```python
from build123d import *

# Parameters (mm, degrees)
BOSS_EXTRUDE1_DEPTH = 508
CUT_EXTRUDE1_DEPTH  = 508
BOSS_EXTRUDE2_DEPTH = 508
BOSS_EXTRUDE3_DEPTH = 635
CUT_EXTRUDE3_DEPTH  = 1016
CUT_EXTRUDE6_DEPTH  = 508
CUT_EXTRUDE7_DEPTH  = 1016
CUT_EXTRUDE8_DEPTH  = 1016
CUT_EXTRUDE9_DEPTH  = 1016
CUT_EXTRUDE10_DEPTH = 2092.737749488
SKETCH11_W          = 6.35
SKETCH11_H          = 822.114235363
BOSS_EXTRUDE4_DEPTH = 76.2
SKETCH12_W          = 6.35
SKETCH12_H          = 1181.577860321
BOSS_EXTRUDE5_DEPTH = 81.28


with BuildPart() as part:
    # Sketch1 → Boss-Extrude1 (new body)
    with BuildSketch(Plane(origin=(0, 0, 0), x_dir=(1, 0, 0), z_dir=(0, 1, 0))):
        Polygon((0, 1066.8), (0, 0), (279.4, 0), (457.2, 1066.8), align=None)
    boss_extrude1 = extrude(amount=BOSS_EXTRUDE1_DEPTH)

    # Sketch2 → Cut-Extrude1 (cut)
    with BuildSketch(Plane.ZY):
        Polygon((0, 0), (-1066.8, 508), (-1066.8, 732.672417782), (0, 732.672417782), align=None)
    cut_extrude1 = extrude(amount=-CUT_EXTRUDE1_DEPTH, mode=Mode.SUBTRACT)

    # Sketch3 → Boss-Extrude2 (add)
    with BuildSketch(Plane.XZ):
        Polygon((0, -1066.8), (0, -1854.2), (609.6, -1854.2), (457.2, -1066.8), align=None)
    boss_extrude2 = extrude(amount=-BOSS_EXTRUDE2_DEPTH)

    # Mirror1: Boss-Extrude1 across plane
    add(boss_extrude1.mirror(Plane(origin=(0, 508, -1066.8), x_dir=(0, 0, 1), z_dir=(1, 0, 0))))

    # Mirror1 2: Cut-Extrude1 across plane
    add(cut_extrude1.mirror(Plane(origin=(0, 508, -1066.8), x_dir=(0, 0, 1), z_dir=(1, 0, 0))), mode=Mode.SUBTRACT)


with BuildPart() as body_2:
    # Sketch4 → Boss-Extrude3 (new body)
    with BuildSketch(Plane.XZ):
        Polygon((279.4, 0), (758.024602406, -943.929756814), (824.163316724, -1854.2), (609.6, -1854.2), (473.605368522, -1854.2), (229.324151542, -858.00394067), align=None)
    boss_extrude3 = extrude(amount=-BOSS_EXTRUDE3_DEPTH)

    # Sketch5 → Cut-Extrude3 (cut)
    with BuildSketch(Plane(origin=(158.02566363, 112.959299077, 80.127753023), x_dir=(-0.31022668993908165, -0.22175505323400505, 0.924437178619848), z_dir=(-0.7520567447205982, -0.5375823192171424, -0.38133437136635806))):
        Polygon((-393.664649125, 703.625608499), (953.241894052, -176.928807588), (-1326.842790058, -923.556364957), (-2274.788319735, -628.326732027), (-2325.528348512, 172.375821483), align=None)
    cut_extrude3 = extrude(amount=-CUT_EXTRUDE3_DEPTH, mode=Mode.SUBTRACT)

    # Sketch6 → Cut-Extrude6 (cut)
    with BuildSketch(Plane(origin=(397.94007399, 254.27896004, 77.020659482), x_dir=(0.13564130705663138, 0.08667317707163243, -0.9869595717131874), z_dir=(0.8316697136780645, 0.5314270256083374, 0.16096833167962543))):
        Polygon((1082.533011894, 1261.854611528), (2538.800510351, 767.688534421), (2437.604130324, -1113.046367909), (306.999460867, -1023.580096849), align=None)
    cut_extrude6 = extrude(amount=CUT_EXTRUDE6_DEPTH, mode=Mode.SUBTRACT)

    # Sketch7 → Cut-Extrude7 (cut)
    with BuildSketch(Plane(origin=(0, 0, 0), x_dir=(1, 0, 0), z_dir=(0, 0.9028605188239303, 0.4299335803923477))):
        Polygon((0, 1181.577860321), (0, 0), (1197.045935399, 0), (1543.879463505, 955.927792479), (976.352766556, 2301.292030359), align=None)
    cut_extrude7 = extrude(amount=CUT_EXTRUDE7_DEPTH, mode=Mode.SUBTRACT)

    # Sketch8 → Cut-Extrude8 (cut)
    with BuildSketch(Plane(origin=(382.681643927, 161.632761359, 74.067414954), x_dir=(0.1616973556962576, 0.06829590736935992, -0.9844742933146776), z_dir=(0.9068988908525647, 0.38304573613058523, 0.1755288175843677))):
        Polygon((1197.556798458, 999.143883777), (2455.295967915, 323.49765858), (2410.705423203, -956.043074474), (776.288597468, -956.043074474), (430.351182168, -503.275200855), align=None)
    cut_extrude8 = extrude(amount=CUT_EXTRUDE8_DEPTH, mode=Mode.SUBTRACT)

    # Sketch9 → Cut-Extrude9 (cut)
    with BuildSketch(Plane(origin=(0, 508, 0), x_dir=(1, 0, 0), z_dir=(0, 1, 0))):
        Polygon((351.522364305, 2301.225932819), (1863.401978722, 1800.09916747), (1313.944223798, 629.194662402), (-286.938271333, 375.015467974), (-444.004316346, 1364.25568729), align=None)
    cut_extrude9 = extrude(amount=CUT_EXTRUDE9_DEPTH, mode=Mode.SUBTRACT)


with BuildPart() as part_1:
    add(part.part)

    # Mirror1 3: Boss-Extrude2, Boss-Extrude3 across plane
    add(boss_extrude2.mirror(Plane(origin=(0, 508, -1066.8), x_dir=(0, 0, 1), z_dir=(1, 0, 0))))
    add(boss_extrude3.mirror(Plane(origin=(0, 508, -1066.8), x_dir=(0, 0, 1), z_dir=(1, 0, 0))))

    # Mirror1 4: Cut-Extrude3, Cut-Extrude6, Cut-Extrude7, Cut-Extrude8, Cut-Extrude9 across plane
    add(cut_extrude3.mirror(Plane(origin=(0, 508, -1066.8), x_dir=(0, 0, 1), z_dir=(1, 0, 0))), mode=Mode.SUBTRACT)
    add(cut_extrude6.mirror(Plane(origin=(0, 508, -1066.8), x_dir=(0, 0, 1), z_dir=(1, 0, 0))), mode=Mode.SUBTRACT)
    add(cut_extrude7.mirror(Plane(origin=(0, 508, -1066.8), x_dir=(0, 0, 1), z_dir=(1, 0, 0))), mode=Mode.SUBTRACT)
    add(cut_extrude8.mirror(Plane(origin=(0, 508, -1066.8), x_dir=(0, 0, 1), z_dir=(1, 0, 0))), mode=Mode.SUBTRACT)
    add(cut_extrude9.mirror(Plane(origin=(0, 508, -1066.8), x_dir=(0, 0, 1), z_dir=(1, 0, 0))), mode=Mode.SUBTRACT)


with BuildPart() as cut_extrude10_tool:
    # Sketch10 → Cut-Extrude10 (new, through all)
    with BuildSketch(Plane(origin=(0, 0, 0), x_dir=(0, 0, -1), z_dir=(1, 0, 0))):
        Polygon((2306.148998717, 875.535830554), (458.236130604, 1137.326156156), (-514.568333215, 141.183628961), (336.70111329, -1596.655316262), (2036.802708671, -1025.71271333), (2740.096775658, -499.622195383), align=None)
    extrude(amount=CUT_EXTRUDE10_DEPTH)


with BuildPart() as part_2:
    add(part_1.part)

    # Cut-Extrude10: cut by cut_extrude10_tool
    add(cut_extrude10_tool.part, mode=Mode.SUBTRACT)

    # Sketch11 → Boss-Extrude4 (add)
    with BuildSketch(Plane(origin=(0, 508, 0), x_dir=(1, 0, 0), z_dir=(0, 1, 0))):
        with Locations((-3.175, 1443.142882319)):
            Rectangle(SKETCH11_W, SKETCH11_H)
    extrude(amount=BOSS_EXTRUDE4_DEPTH)

    # Sketch12 → Boss-Extrude5 (add)
    with BuildSketch(Plane(origin=(0, 0, 0), x_dir=(1, 0, 0), z_dir=(0, 0.9028605188239304, 0.42993358039234775))):
        with Locations((-3.175, 590.788930161)):
            Rectangle(SKETCH12_W, SKETCH12_H)
    extrude(amount=BOSS_EXTRUDE5_DEPTH)


with BuildPart() as body_2_1:
    add(body_2.part)

    # Cut-Extrude10: cut by cut_extrude10_tool
    add(cut_extrude10_tool.part, mode=Mode.SUBTRACT)


solid = part_2.part
```
Geometry: final body of the model. Coordinates: model frame, mm. A direction names the side the tool comes from. Round coordinates to 2 decimals unless told otherwise and drop trailing zeros. Write each loop counter-clockwise with the first axis right and the second up, starting at its lowest first coordinate (ties: lowest second). Pieces come first, ordered by that corner, then holes. Notation, with made-up numbers: M 64,23 L 97,23 A21 ccw 97,37 Z; hole C 66.5,5 d5. An arc over 180 degrees is marked long. Answer in a Markdown table with one row per item. Add a question column.
(1) Cut plane C-C, the plane x = -66.5. Return the cut outline in (y, z), then the cut area to 3 significant figures.
(2) Cut plane B-B, the plane z = -921.5. Return the cut outline in (x, y).
(3) Ray query, L1, parallel to X at y = 325.5, z = -515; L2, parallel to Y at x = -494.5, z = -1747.5; L3, parallel to Y at x = -463.5, z = -602. Return the intervals inside material, ascending.
(4) Cut plane D-D, the plane z = -338. Return the cut outline in (x, y).
(5) Cut plane A-A, the plane y = 251. Return the cut outline in (x, z).
(6) Contact query for flat-ended pins moving along their axis: pin 1 (1 mm diameter, centred on x = -157.5, y = 169, fed in from +Z); pin 2 (12 mm diameter, centred on y = 306.5, z = -1190, fed in from -X); pin 3 (4 mm diameter, centred on x = -304, z = -450, fed in from +Y). Output: stop coordinate, or through.
(7) Reachability of faces 1 (the face through (-245, 508, -1466)), 2 (the face through (0, 261, -1164)), 3 (the face through (-6.35, 437, -853)) from +Z, -Z, +X, -X, +Y, -Y: full face, straight path, thin tool, end or side. Return the list, or none.
Established:
| question | item | result |
|---|---|---|
| 1 | outline | M 0,-1854.2 L 508,-1854.2 L 508,-1066.8 L 0,0 Z |
| 1 | area | 671,000 mm² |
| 2 | outline | M -643.64,0 L 0,0 L 0,528.83 L -6.35,528.83 L -6.35,438.81 L -432.98,438.81 L -494.87,352.24 Z |
| 3 | L1 | -6.35 to 0 |
| 3 | L2 | 0 to 508 |
| 3 | L3 | 0 to 169.48 |
| 4 | outline | M -450.78,0 L 0,0 L 0,250.98 L -6.35,250.98 L -6.35,160.95 L -335.73,160.95 Z |
| 5 | outline | M -718.15,-1854.2 L 0,-1854.2 L 0,-338.05 L -6.35,-338.05 L -6.35,-527.1 L -367.25,-527.1 L -519.35,-827.06 Z |
| 6 | pin 1 | z = -353.85 |
| 6 | pin 2 | x = -568.94 |
| 6 | pin 3 | y = 215.24 |
| 7 | face 1 | +Z, -Z, -X, +Y |
| 7 | face 2 | +Z, -Z, +X, +Y, -Y |
| 7 | face 3 | +Z, -X, +Y |
